```python
from build123d import *

# Parameters (mm, degrees)
SKETCH1_R            = 35
BOSS_EXTRUDE1_DEPTH  = 10
SKETCH2_R            = 23.5
BOSS_EXTRUDE2_DEPTH  = 13
BOSS_EXTRUDE4_DEPTH  = 4
SKETCH5_R            = 1.5
CUT_EXTRUDE1_DEPTH   = 86.86350209
SKETCH6_W            = 4
SKETCH6_H            = 9
BOSS_EXTRUDE5_DEPTH  = 3
FILLET1_R            = 2
FILLET1_OF_MIRROR2_R = 2
SKETCH8_R            = 10
CUT_EXTRUDE2_DEPTH   = 10
SKETCH11_W           = 10.23491337
SKETCH11_H           = 17.961461559
BOSS_EXTRUDE6_DEPTH  = 3


with BuildPart() as part:
    # Sketch1 → Boss-Extrude1 (new body)
    with BuildSketch(Plane(origin=(0, 0, 0), x_dir=(0, 0, -1), z_dir=(1, 0, 0))):
        Circle(SKETCH1_R)
    extrude(amount=BOSS_EXTRUDE1_DEPTH)

    # Sketch2 → Boss-Extrude2 (add)
    with BuildSketch(Plane(origin=(10, 0, 0), x_dir=(0, 0, -1), z_dir=(1, 0, 0))):
        with Locations(Location((0, 0, 0), (0, 0, 180))):
            Circle(SKETCH2_R)
    extrude(amount=BOSS_EXTRUDE2_DEPTH)

    # Sketch3 → Boss-Extrude4 (add)
    with BuildSketch(Plane(origin=(0, 13, 0), x_dir=(1, 0, 0), z_dir=(0, 1, 0))):
        Polygon((23, 35), (23, -35), (30.392057511, -43.809511096), (35.392057511, -43.809511096), (52.43346001, -23.500358445), (52.43346001, 23.500358445), (35.392057511, 43.809511096), (30.392057511, 43.809511096), align=None)
    boss_extrude4 = extrude(amount=BOSS_EXTRUDE4_DEPTH)

    # Sketch5 → Cut-Extrude1 (cut, symmetric)
    with BuildSketch(Plane(origin=(0, 17, 0), x_dir=(1, 0, 0), z_dir=(0, 1, 0))):
        with Locations(Location((32.892057511, -40.809511096, 0), (0, 0, 270))):
            Circle(SKETCH5_R)
        with Locations(Location((32.892057511, 40.809511096, 0), (0, 0, 270))):
            Circle(SKETCH5_R)
    cut_extrude1 = extrude(amount=CUT_EXTRUDE1_DEPTH, both=True, mode=Mode.SUBTRACT)

    # Sketch6 → Boss-Extrude5 (add)
    with BuildSketch(Plane(origin=(23, 0, 0), x_dir=(0, 0, -1), z_dir=(1, 0, 0))):
        with Locations((0, 21.5)):
            Rectangle(SKETCH6_W, SKETCH6_H)
    boss_extrude5 = extrude(amount=BOSS_EXTRUDE5_DEPTH)

    # Fillet1
    fillet1_edges = [part.edges().sort_by_distance(p)[0] for p in [
        (24.5, 26, -2),
        (24.5, 26, 2),
    ]]
    fillet(fillet1_edges, radius=FILLET1_R - 0.0001)  # a hair under: the kernel refuses the full size

    # Mirror2: Boss-Extrude5 across plane
    add(boss_extrude5.mirror(Plane.ZX))

    # Fillet1 of Mirror2
    fillet1_of_mirror2_edges = [part.edges().sort_by_distance(p)[0] for p in [
        (24.5, -26, -2),
        (24.5, -26, 2),
    ]]
    fillet(fillet1_of_mirror2_edges, radius=FILLET1_OF_MIRROR2_R - 0.0001)  # a hair under: the kernel refuses the full size

    # Sketch8 → Cut-Extrude2 (cut)
    with BuildSketch(Plane.ZY):
        Circle(SKETCH8_R)
    extrude(amount=-CUT_EXTRUDE2_DEPTH, mode=Mode.SUBTRACT)

    # Mirror3: Boss-Extrude4, Cut-Extrude1 across plane
    add(boss_extrude4.mirror(Plane(origin=(0, 8, 0), x_dir=(0, 0, 1), z_dir=(0, -1, 0))))
    add(cut_extrude1.mirror(Plane(origin=(0, 8, 0), x_dir=(0, 0, 1), z_dir=(0, -1, 0))), mode=Mode.SUBTRACT)

    # Sketch11 → Boss-Extrude6 (add)
    with BuildSketch(Plane(origin=(52.43346001, 0, 0), x_dir=(0, 0, -1), z_dir=(1, 0, 0))):
        with Locations((0, 8.019269221)):
            Rectangle(SKETCH11_W, SKETCH11_H)
    extrude(amount=BOSS_EXTRUDE6_DEPTH)


solid = part.part
```
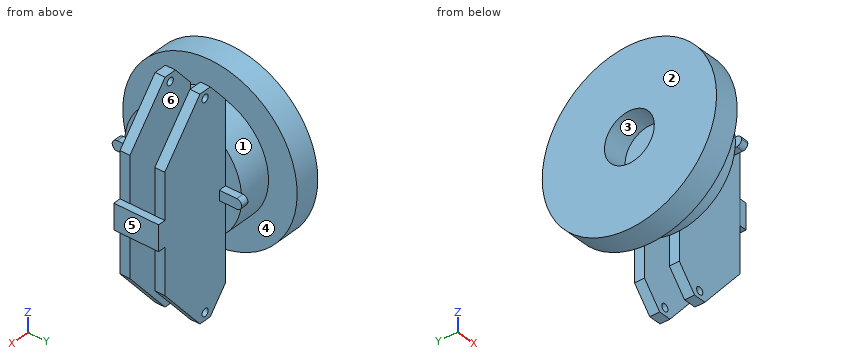
Input: part model. Units: mm. Frame: model coordinates. Face numbers are marked on the shaded views. A direction names the side the tool comes from. Round coordinates to 2 decimals unless told otherwise and drop trailing zeros. Loops run counter-clockwise (first coordinate to the right, second up) from the corner with the lowest first, then second, coordinate; pieces in that order, holes last.
1) Material intervals for line 1 (Y direction, x = 33, z = 33.5); line 2 (Y direction, x = 2, z = 0); line 3 (X direction, y = 9, z = 14), sorted ascending.
Ans:
line 1: y = -1 to 3, 13 to 17
line 2: y = -35 to -10, 10 to 35
line 3: x = 0 to 23
2) Set-up query: the marked faces 4, 5 and 6. Return all of +Z, -Z, +X, -X, +Y, -Y with unobstructed straight access to the full face (end or side cutting, diameter ignored); none if empty.
Ans:
face 4: none
face 5: +Z, -Z, +X, +Y, -Y
face 6: +Z, -Z
3) Pull-direction query (Y, two-part tool) for the marked faces 1, 2 and 3; classes: released by +Y, released by -Y, zero draft, split by the parting line, or undercut.
Ans:
face 1: split by the parting line
face 2: zero draft
face 3: undercut
4) Section query A-A on z = -30.5. Return the cut outline in (x, y), plus the area to 3 significant figures.
Ans:
outline: (0, -17.17) - (10, -17.17) - (10, 17.17) - (0, 17.17) - close; (23, -1) - (46.56, -1) - (46.56, 3) - (23, 3) - close; (23, 13) - (46.56, 13) - (46.56, 17) - (23, 17) - close
area: 532 mm2
5) Pin query (flat end, axial travel): pin 1 (11 mm diameter, centred on y = -9.5, z = 0.5, fed in from +X); pin 2 (2 mm diameter, centred on y = -24, z = 29, fed in from +X); pin 3 (3 mm diameter, centred on y = 15, z = -18, fed in from +X); pin 4 (1.2 mm diameter, centred on y = -23, z = 1, fed in from +X). Return the tip coordinate at first contact, or that it passes through.
Ans:
pin 1: stops at x = 23
pin 2: passes through
pin 3: stops at x = 52.43
pin 4: stops at x = 26
6) Section query B-B on x = 20.5. Return the cut outline in (y, z), plus the area to 3 significant figures.
Ans:
outline: circle Ø47 at (0, 0)
area: 1,730 mm2
